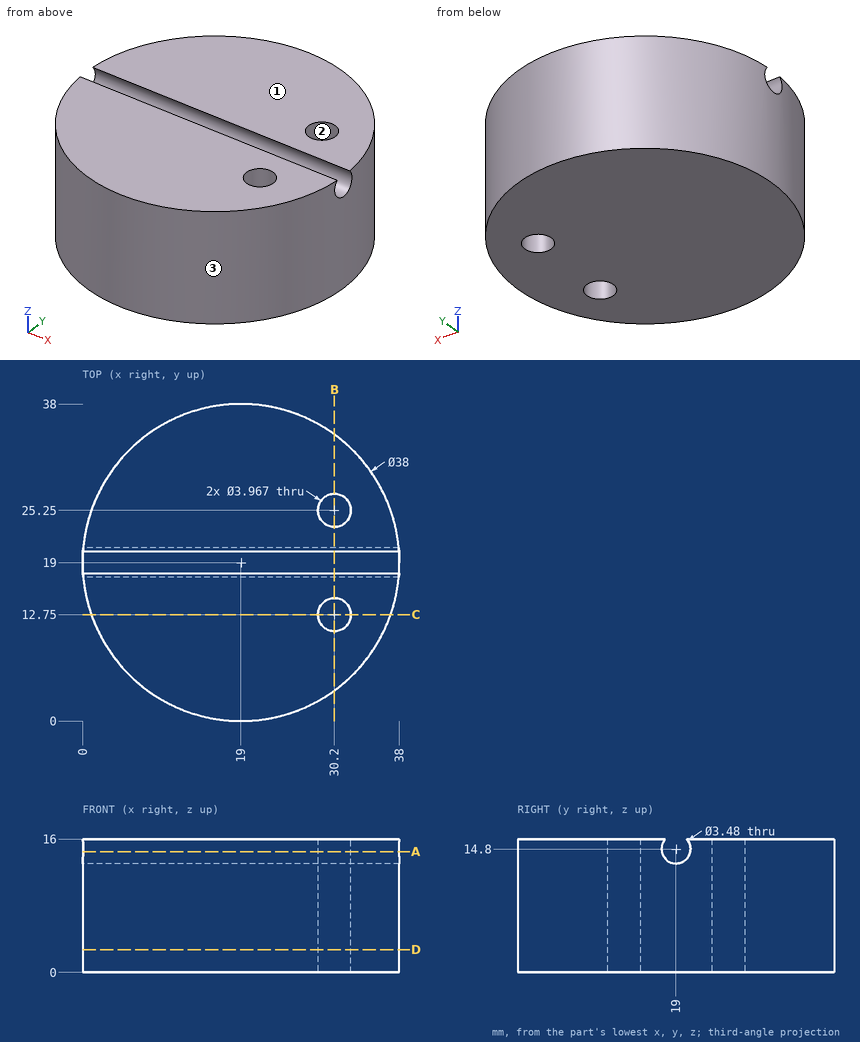
Design review of the part shown in the three views and the two pictorial views. Dimensions are in mm from the part's minimum x, y and z. Give positions to 0.01 mm unless a question says otherwise; leave off trailing zeros. Write each loop counter-clockwise with the first axis right and the second up, starting at its lowest first coordinate (ties: lowest second). Pieces come first, ordered by that corner, then holes. Notation, with made-up numbers: M 45.25,8 L 83.25,8 A9 cw 83.25,18 Z; hole C -34,60.25 d9. An arc over 180 degrees is marked long. Answer as CSV lines item,"result".
1. Consider section C-C, the plane y = 12.75. Write out the cut boundary in (x, z), then the cut area to 3 significant figures.
Findings:
outline,"M 1.06,0 L 28.22,0 L 28.22,16 L 1.06,16 Z; M 32.18,0 L 36.94,0 L 36.94,16 L 32.18,16 Z"
area,"511 mm2"
2. Consider section D-D, the plane z = 2.75. Write out the cut boundary in (x, y).
Findings:
outline,"C 19,19 d38; hole C 30.2,12.75 d3.97; hole C 30.2,25.25 d3.97"
3. Draft analysis for pull direction X (two halves, no side actions). For the marked faces 1, 2 and 3, state which applies: +X half, -X half, draft (parallel to the pull), parting line (faces both ways), or undercut.
Findings:
face 1,"draft"
face 2,"undercut"
face 3,"parting line"
4. For pin 1 (2 mm diameter, centred on x = 22.5, z = 4.5, fed in from -Y); pin 2 (8 mm diameter, centred on x = 15, z = 8.5, fed in from +Y); pin 3 (4 mm diameter, centred on x = 11, z = 3.5, fed in from -Y), all flat-tipped, find the tip position at first contact; note any pin that passes through.
Findings:
pin 1,"stops at y = 0.17"
pin 2,"stops at y = 38"
pin 3,"stops at y = 0.97"
5. Wall thickness on line 1 (Y direction, x = 30, z = 6.25); line 2 (Y direction, x = 30.2, z = 7.25); line 3 (Z direction, x = 17, y = 19): over which ranges is each line inside the solid? List them lowest first.
Findings:
line 1,"y = 3.51 to 10.78, 14.72 to 23.28, 27.22 to 34.49"
line 2,"y = 3.65 to 10.77, 14.73 to 23.27, 27.23 to 34.35"
line 3,"z = 0 to 13.06"
6. Consider section A-A, the plane z = 14.5. Write out the cut boundary in (x, y).
Findings:
outline,"M 0.08,17.29 A19 ccw 37.92,17.29 Z; M 0.08,20.71 L 37.92,20.71 A19 ccw Z; hole C 30.2,12.75 d3.97; hole C 30.2,25.25 d3.97"
7. Consider section B-B, the plane x = 30.2. Write out the cut boundary in (y, z).
Findings:
outline,"M 3.65,0 L 10.77,0 L 10.77,16 L 3.65,16 Z; M 14.73,0 L 23.27,0 L 23.27,16 L 20.26,16 A1.74 cw long 17.74,16 L 14.73,16 Z; M 27.23,0 L 34.35,0 L 34.35,16 L 27.23,16 Z"
